```python
from build123d import *

# Parameters (mm, degrees)
SKETCH1_R           = 4.5
SKETCH1_R_2         = 4
BOSS_EXTRUDE1_DEPTH = 5
SKETCH1_5_R         = 4
CUT_EXTRUDE2_DEPTH  = 13.737739203
SKETCH1_6_R         = 4.5
SKETCH1_6_R_2       = 4
BOSS_EXTRUDE4_DEPTH = 10
SKETCH3_R           = 5
BOSS_EXTRUDE5_DEPTH = 5
SKETCH4_R           = 4.5
BOSS_EXTRUDE6_DEPTH = 5
SKETCH5_R           = 5
BOSS_EXTRUDE7_DEPTH = 5
SKETCH6_R           = 3.5
CUT_EXTRUDE3_DEPTH  = 5


with BuildPart() as part:
    # Sketch1 → Boss-Extrude1 (new body)
    # profile 1 of 5: a face of its own
    with BuildSketch(Plane(origin=(0, 0, 0), x_dir=(1, 0, 0), z_dir=(0, 1, 0))):
        with BuildLine():
            Line((-8, -7.5), (8, -7.5))
            ThreePointArc((8, -7.5), (8.707106781, -7.207106781), (9, -6.5))
            Line((9, -6.5), (9, 6.5))
            ThreePointArc((9, 6.5), (8.707106781, 7.207106781), (8, 7.5))
            Line((8, 7.5), (-8, 7.5))
            ThreePointArc((-8, 7.5), (-8.707106781, 7.207106781), (-9, 6.5))
            Line((-9, 6.5), (-9, -6.5))
            ThreePointArc((-9, -6.5), (-8.707106781, -7.207106781), (-8, -7.5))
        make_face()
        Circle(SKETCH1_R, mode=Mode.SUBTRACT)
        with BuildLine():
            Line((4.5, -5), (4.5, 5))
            ThreePointArc((4.5, 5), (6, 6.5), (7.5, 5))
            Line((7.5, 5), (7.5, -5))
            ThreePointArc((7.5, -5), (6, -6.5), (4.5, -5))
        make_face(mode=Mode.SUBTRACT)
        with BuildLine():
            Line((-4.5, -5), (-4.5, 5))
            ThreePointArc((-4.5, 5), (-6, 6.5), (-7.5, 5))
            Line((-7.5, 5), (-7.5, -5))
            ThreePointArc((-7.5, -5), (-6, -6.5), (-4.5, -5))
        make_face(mode=Mode.SUBTRACT)
    # profile 2 of 5: a face of its own
    with BuildSketch(Plane(origin=(0, 0, 0), x_dir=(1, 0, 0), z_dir=(0, 1, 0))):
        with BuildLine():
            ThreePointArc((-7.5, 5), (-6, 6.5), (-4.5, 5))
            Line((-4.5, 5), (-4.5, -5))
            ThreePointArc((-4.5, -5), (-6, -6.5), (-7.5, -5))
            Line((-7.5, -5), (-7.5, 5))
        make_face()
    # profile 3 of 5: a face of its own
    with BuildSketch(Plane(origin=(0, 0, 0), x_dir=(1, 0, 0), z_dir=(0, 1, 0))):
        Circle(SKETCH1_R)
        Circle(SKETCH1_R_2, mode=Mode.SUBTRACT)
    # profile 4 of 5: a face of its own
    with BuildSketch(Plane(origin=(0, 0, 0), x_dir=(1, 0, 0), z_dir=(0, 1, 0))):
        Circle(SKETCH1_R_2)
    # profile 5 of 5: a face of its own
    with BuildSketch(Plane(origin=(0, 0, 0), x_dir=(1, 0, 0), z_dir=(0, 1, 0))):
        with BuildLine():
            Line((7.5, -5), (7.5, 5))
            ThreePointArc((7.5, 5), (6, 6.5), (4.5, 5))
            Line((4.5, 5), (4.5, -5))
            ThreePointArc((4.5, -5), (6, -6.5), (7.5, -5))
        make_face()
    extrude(amount=BOSS_EXTRUDE1_DEPTH)

    # Sketch1<5> → Cut-Extrude2 (cut, through all)
    with BuildSketch(Plane(origin=(0, 0, 0), x_dir=(1, 0, 0), z_dir=(0, 1, 0))):
        with Locations(Location((0, 0, 0), (0, 0, 270))):
            Circle(SKETCH1_5_R)
    extrude(amount=CUT_EXTRUDE2_DEPTH, mode=Mode.SUBTRACT)

    # Sketch1<6> → Boss-Extrude4 (add)
    with BuildSketch(Plane(origin=(0, 0, 0), x_dir=(1, 0, 0), z_dir=(0, 1, 0))):
        with Locations(Location((0, 0, 0), (0, 0, 270))):
            Circle(SKETCH1_6_R)
        with Locations(Location((0, 0, 0), (0, 0, 270))):
            Circle(SKETCH1_6_R_2, mode=Mode.SUBTRACT)
    extrude(amount=BOSS_EXTRUDE4_DEPTH)

    # Sketch3 → Boss-Extrude5 (add)
    with BuildSketch(Plane(origin=(0, 10, 0), x_dir=(1, 0, 0), z_dir=(0, 1, 0))):
        with Locations(Location((0, 0, 0), (0, 0, 270))):
            Circle(SKETCH3_R)
    extrude(amount=BOSS_EXTRUDE5_DEPTH)

    # Sketch4 → Boss-Extrude6 (add)
    with BuildSketch(Plane(origin=(0, 15, 0), x_dir=(1, 0, 0), z_dir=(0, 1, 0))):
        with Locations(Location((0, 0, 0), (0, 0, 270))):
            Circle(SKETCH4_R)
    extrude(amount=BOSS_EXTRUDE6_DEPTH)

    # Sketch5 → Boss-Extrude7 (add)
    with BuildSketch(Plane(origin=(0, 20, 0), x_dir=(1, 0, 0), z_dir=(0, 1, 0))):
        with Locations(Location((0, 0, 0), (0, 0, 270))):
            Circle(SKETCH5_R)
    extrude(amount=BOSS_EXTRUDE7_DEPTH)

    # Sketch6 → Cut-Extrude3 (cut)
    with BuildSketch(Plane(origin=(0, 25, 0), x_dir=(1, 0, 0), z_dir=(0, 1, 0))):
        with Locations(Location((0, 0, 0), (0, 0, 270))):
            Circle(SKETCH6_R)
    extrude(amount=-CUT_EXTRUDE3_DEPTH, mode=Mode.SUBTRACT)


solid = part.part
```
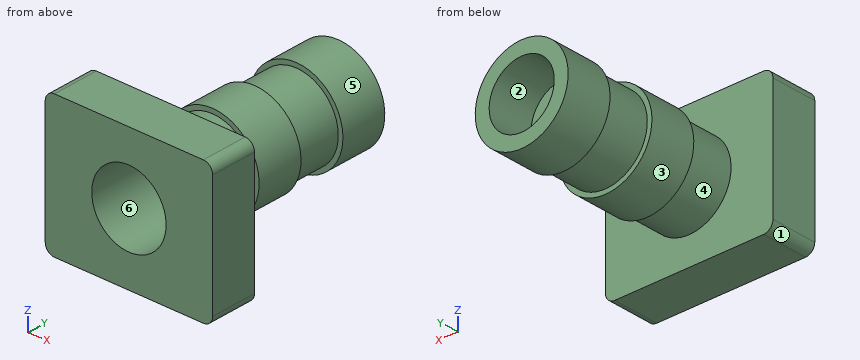
The listing builds one solid part. Answer for the finished solid, in the listing's coordinates (mm). Face numbers are marked on the shaded views. A direction names the side the tool comes from. Coordinates: 2 decimals unless noted, no trailing zeros. Write each loop counter-clockwise with the first axis right and the second up, starting at its lowest first coordinate (ties: lowest second). Pieces come first, ordered by that corner, then holes. Notation, with made-up numbers: M -32.5,-9 L 21.5,-9 A18 ccw 21.5,19 Z; hole C -31,76.5 d2. An arc over 180 degrees is marked long. Use a Markdown table: item, result. Add a question column.
1. Section C-C (x = 0) is taken. Give the vertices of the cut face in (y, z).
2. Section D-D (x = -5.5) is taken. Give the vertices of the cut face in (y, z), plus the area to 3 significant figures.
3. For a pull along X with two mould halves and no side action, classify the marked faces 1, 2 and 3 as +X half, -X half, draft (parallel to the pull), parting line (faces both ways), or undercut.
4. Which of the six approach directions +Z, -Z, +X, -X, +Y, -Y give full straight-line access (tool end or side, diameter ignored) to the marked faces 4, 5 and 6?
5. Section B-B (y = 22.25) is taken. Give the vertices of the cut face in (x, z), plus the area to 3 significant figures.
6. Section A-A (z = 0) is taken. Give the vertices of the cut face in (x, y), plus the area to 3 significant figures.
7. Straight lines are drawn through the part: line 1 along X through (y, z) = (21.75, 0); line 2 along Y through (x, z) = (3.75, 3); line 3 along X through (y, z) = (2.75, 0). For each, find the intervals that lie inside material, in ascending order. Write a range as [from, to].
8. Given P1, Ø8, axis at x = 2, z = -1.5, coming from the -Y side; P2, Ø3, axis at x = 0.5, z = 1.5, coming from the +Y side; P3, Ø6.5, axis at x = 0, z = 0, coming from the -Y side; P4, Ø1.5, axis at x = 2, y = 21.5, coming from the +Z side, each flat-ended and moving along its own axis, determine where each tip first touches the part or whether it passes through.
Data:
| question | item | result |
|---|---|---|
| 1 | outline | M 0,-7.5 L 5,-7.5 L 5,-4.5 L 10,-4.5 L 10,-5 L 15,-5 L 15,-4.5 L 20,-4.5 L 20,-5 L 25,-5 L 25,-3.5 L 20,-3.5 L 20,3.5 L 25,3.5 L 25,5 L 20,5 L 20,4.5 L 15,4.5 L 15,5 L 10,5 L 10,4.5 L 5,4.5 L 5,7.5 L 0,7.5 L 0,4 L 10,4 L 10,-4 L 0,-4 Z |
| 2 | outline | M 0,-7.5 L 5,-7.5 L 5,7.5 L 0,7.5 Z |
| 2 | area | 75.0 mm2 |
| 3 | face 1 | -X half |
| 3 | face 2 | undercut |
| 3 | face 3 | parting line |
| 4 | face 4 | none |
| 4 | face 5 | +Y |
| 4 | face 6 | -Y |
| 5 | outline | C 0,0 d10; hole C 0,0 d7 |
| 5 | area | 40.1 mm2 |
| 6 | outline | M -9,0 L -4,0 L -4,10 L 4,10 L 4,0 L 9,0 L 9,5 L 4.5,5 L 4.5,10 L 5,10 L 5,15 L 4.5,15 L 4.5,20 L 5,20 L 5,25 L 3.5,25 L 3.5,20 L -3.5,20 L -3.5,25 L -5,25 L -5,20 L -4.5,20 L -4.5,15 L -5,15 L -5,10 L -4.5,10 L -4.5,5 L -9,5 Z |
| 6 | area | 165 mm2 |
| 7 | line 1 | x = [-5, -3.5], [3.5, 5] |
| 7 | line 2 | y = [0, 5], [10, 15], [20, 25] |
| 7 | line 3 | x = [-9, -4], [4, 9] |
| 8 | P1 | stops at y = 0 |
| 8 | P2 | stops at y = 20 |
| 8 | P3 | stops at y = 10 |
| 8 | P4 | stops at z = 4.84 |
